from build123d import *


with BuildPart() as part:
    # 草图2 → 旋转2 (revolve)
    with BuildSketch(Plane(origin=(0, 0, 0), x_dir=(0, 0, -1), z_dir=(1, 0, 0)), mode=Mode.PRIVATE) as revolve_2_sk:
        Polygon((0, 60), (0, 57), (3, 57), (13.416437738, 57), (21.516437738, 3), (21.966437738, 0), (25, 0), (16, 60), align=None)
        Polygon((5, 3), (5, 0), (21.966437738, 0), (21.516437738, 3), align=None)
    revolve(revolve_2_sk.sketch.rotate(Axis((0, 60, 0), (0, -1, 0)), 180), axis=Axis((0, 60, 0), (0, -1, 0)))


solid = part.part
Source: CAD feature listing. Evaluate the final solid. Frame: model axes, mm. A direction names the side the tool comes from. Give positions to 0.01 mm unless a question says otherwise; leave off trailing zeros. Write each loop counter-clockwise with the first axis right and the second up, starting at its lowest first coordinate (ties: lowest second). Pieces come first, ordered by that corner, then holes. Notation, with made-up numbers: (24, 75) -> (75, 75) arc R21 cw to (75, 85) -> close; hole circle Ø8 at (-10, 51). An arc over 180 degrees is marked (long way). Return JSON: item names as keys, results as strings. Group by question number.
1. Mould query, pull axis Z, two halves, no side actions, for faces 3 (the face through (4, 3, 4)), 4 (the face through (0, 1, -5)), 5 (the face through (-6.139, 30.42, 19.493)), 6 (the face through (0, 60, 0)). Classes: +Z half, -Z half, draft (parallel to the pull), parting line (faces both ways), or undercut.
2. Material intervals for line 1 (Y direction, x = 12, z = -5); line 2 (Z direction, x = 19, y = 5); line 3 (X direction, y = 1.6, z = 0), sorted ascending. Write a range as from..to.
3. Pin query (flat end, axial travel): pin 1 Ø8 at (x, y) = (18, 17) entering from +Z; pin 2 Ø4 at (x, y) = (6, 27.5) entering from -Z; pin 3 Ø12 at (x, z) = (16, 15.5) entering from -Y; pin 4 Ø1 at (y, z) = (23, 12) entering from -X. Return the tip coordinate at first contact, or that it passes through.
4. Section C-C, the plane y = 16.5. Output: boundary loops of the cut face in (x, z) (3 decimals), then the cut area to 3 significant figures.
5. Section A-A, the plane z = 0. Output: boundary loops of the cut face in (x, y).
6. Section B-B, the plane y = 25.5. Output: boundary loops of the cut face in (x, z) (3 decimals).
7. Access query for faces 1 (the face through (0, 57, 0)), 2 (the face through (5.2, 0, 0.3)). Directions: +Z, -Z, +X, -X, +Y, -Y. A direction counts if a zero-diameter tool reaches every point of the face in a straight line with its end or side. Return the directions, or none.
Determined:
{
 "1": {"face 3": "undercut", "face 4": "undercut", "face 5": "parting line", "face 6": "draft"},
 "2": {"line 1": "y = 0..3, 57..60", "line 2": "z = -15.07..-9.44, 9.44..15.07", "line 3": "x = -24.76..-5, 5..24.76"},
 "3": {"pin 1": "stops at z = 17.64", "pin 2": "stops at z = -20.59", "pin 3": "stops at y = 0", "pin 4": "stops at x = -18.24"},
 "4": {"outline": "circle Ø45.05 at (0, 0); hole circle Ø38.983 at (0, 0)", "area": "400 mm2"},
 "5": {"outline": "(-25, 0) -> (-5, 0) -> (-5, 3) -> (-21.52, 3) -> (-13.42, 57) -> (13.42, 57) -> (21.52, 3) -> (5, 3) -> (5, 0) -> (25, 0) -> (16, 60) -> (-16, 60) -> close"},
 "6": {"outline": "circle Ø42.35 at (0, 0); hole circle Ø36.283 at (0, 0)"},
 "7": {"face 1": "none", "face 2": "+Z, -Z, +X, -X, -Y"}
}
